from build123d import *

# Parameters (mm, degrees)
SKETCH1_W             = 198
SKETCH1_H             = 108
BOSS_EXTRUDE1_DEPTH   = 40
SKETCH4_W             = 181
SKETCH4_H             = 45
CUT_EXTRUDE2_DEPTH    = 10
CUT_EXTRUDE3_DEPTH    = 175
BOSS_EXTRUDE11_DEPTH  = 10
CUT_EXTRUDE12_DEPTH   = 175
CUT_EXTRUDE28_DEPTH   = 14.5
CUT_EXTRUDE29_DEPTH   = 14.5
CUT_EXTRUDE40_REACH   = 231.059
CUT_EXTRUDE5_DEPTH    = 23
SKETCH12_R            = 3.15
CUT_EXTRUDE9_DEPTH    = 230.058944379
SKETCH13_R            = 4.5
CUT_EXTRUDE10_DEPTH   = 16.5
SKETCH14_R            = 4.5
CUT_EXTRUDE11_DEPTH   = 16.5
SKETCH41_R            = 2.9
CUT_EXTRUDE21_DEPTH   = 7
CUT_EXTRUDE22_DEPTH   = 10
CUT_EXTRUDE23_DEPTH   = 10
CUT_EXTRUDE32_DEPTH   = 43.3
CUT_EXTRUDE34_DEPTH   = 55.4
CUT_EXTRUDE36_DEPTH   = 55.4
SKETCH90_R            = 6.1
CUT_EXTRUDE38_DEPTH   = 17
SKETCH96_R            = 2
CUT_EXTRUDE39_DEPTH   = 230.058944379
SKETCH98_R            = 7.5
CUT_EXTRUDE41_DEPTH   = 4
CORTAR_EXTRUIR1_DEPTH = 23
CORTAR_EXTRUIR2_DEPTH = 23


with BuildPart() as part:
    # Sketch1 → Boss-Extrude1 (new body)
    with BuildSketch(Plane(origin=(0, 0, 0), x_dir=(1, 0, 0), z_dir=(0, 1, 0))):
        with Locations((99, 54)):
            Rectangle(SKETCH1_W, SKETCH1_H)
    extrude(amount=BOSS_EXTRUDE1_DEPTH)

    # Sketch4 → Cut-Extrude2 (cut)
    with BuildSketch(Plane(origin=(0, 0, 0), x_dir=(1, 0, 0), z_dir=(0, 1, 0))):
        with Locations((99, 54)):
            Rectangle(SKETCH4_W, SKETCH4_H)
    extrude(amount=CUT_EXTRUDE2_DEPTH, mode=Mode.SUBTRACT)

    # Sketch5 → Cut-Extrude3 (cut)
    with BuildSketch(Plane(origin=(198, 0, 0), x_dir=(0, 0, -1), z_dir=(1, 0, 0))):
        Polygon((54, 40), (108, 28.52194567), (108, 40), align=None)
    extrude(amount=-CUT_EXTRUDE3_DEPTH, mode=Mode.SUBTRACT)

    # Sketch53 → Boss-Extrude11 (add)
    with BuildSketch(Plane(origin=(0, 10, 0), x_dir=(-1, 0, 0), z_dir=(0, -1, 0))):
        Polygon((-8.5, 51.5), (-8.5, 31.5), (-39.5, 31.5), align=None)
        Polygon((-8.5, 56.5), (-8.5, 76.5), (-39.5, 76.5), align=None)
        Polygon((-158.5, 76.5), (-189.5, 56.5), (-189.5, 76.5), align=None)
        Polygon((-158.5, 31.5), (-189.5, 51.5), (-189.5, 31.5), align=None)
    extrude(amount=BOSS_EXTRUDE11_DEPTH)

    # Sketch18 → Cut-Extrude12 (cut)
    with BuildSketch(Plane(origin=(198, 0, 0), x_dir=(0, 0, -1), z_dir=(1, 0, 0))):
        Polygon((0, 28.915391904), (0, 40), (54, 40), align=None)
    extrude(amount=-CUT_EXTRUDE12_DEPTH, mode=Mode.SUBTRACT)

    # Izq → Cut-Extrude28 (cut)
    with BuildSketch(Plane(origin=(0, 28.012686094, -12.204810084), x_dir=(1, 0, 0), z_dir=(0, 0.9167660546215654, -0.3994245874925693))):
        Polygon((8.5, 48.862182113), (29.5, 70.132603179), (8.5, 70.132603179), align=None)
    cut_extrude28 = extrude(amount=-CUT_EXTRUDE28_DEPTH, mode=Mode.SUBTRACT)

    # Der → Cut-Extrude29 (cut)
    with BuildSketch(Plane(origin=(0, -11.144923858, -4.62106599), x_dir=(1, 0, 0), z_dir=(0, 0.9237421135716327, 0.38301502270043264))):
        Polygon((8.5, 51.290217599), (29.5, 29.097876578), (8.5, 29.097876578), align=None)
    cut_extrude29 = extrude(amount=-CUT_EXTRUDE29_DEPTH, mode=Mode.SUBTRACT)

    # Cut-Extrude40: up to this face of the body (flat: up to its plane)
    cut_extrude40_end = Plane(part.part.faces().sort_by_distance((99, 10, -54))[0])
    # Sketch97 → Cut-Extrude40 (cut, up to the picked face)
    with BuildSketch(Plane(origin=(0, 0, 0), x_dir=(1, 0, 0), z_dir=(0, 1, 0)), mode=Mode.PRIVATE) as cut_extrude40_sk1:
        Polygon((8.5, 57.5), (29.5, 76.5), (158.5, 76.5), (189.5, 56.5), (189.5, 51.5), (158.5, 31.5), (29.5, 31.5), (8.5, 51.5), align=None)
    cut_extrude40_tool1 = split(extrude(cut_extrude40_sk1.sketch, amount=CUT_EXTRUDE40_REACH, mode=Mode.PRIVATE), bisect_by=cut_extrude40_end, keep=Keep.BOTH, mode=Mode.PRIVATE)
    cut_extrude40 = cut_extrude40_tool1.solids().sort_by(Axis((96.82024, 0, -54.014019), (0, 1, 0)))[0]
    add(cut_extrude40, mode=Mode.SUBTRACT)

    # Mirror2: Cut-Extrude28, Cut-Extrude29, Cut-Extrude40 across plane
    add(cut_extrude28.mirror(Plane(origin=(99, 0, 0), x_dir=(0, 0, 1), z_dir=(1, 0, 0))), mode=Mode.SUBTRACT)
    add(cut_extrude29.mirror(Plane(origin=(99, 0, 0), x_dir=(0, 0, 1), z_dir=(1, 0, 0))), mode=Mode.SUBTRACT)
    add(cut_extrude40.mirror(Plane(origin=(99, 0, 0), x_dir=(0, 0, 1), z_dir=(1, 0, 0))), mode=Mode.SUBTRACT)

    # Sketch7 → Cut-Extrude5 (cut)
    with BuildSketch(Plane(origin=(0, 0, 0), x_dir=(0, 0, -1), z_dir=(1, 0, 0))):
        Polygon((108, 40), (108, 35), (83.505102572, 40), align=None)
        Polygon((0, 35), (0, 40), (24.494897428, 40), align=None)
    extrude(amount=CUT_EXTRUDE5_DEPTH, mode=Mode.SUBTRACT)

    # Sketch12 → Cut-Extrude9 (cut, through all)
    with BuildSketch(Plane(origin=(0, 40, 0), x_dir=(1, 0, 0), z_dir=(0, 1, 0))):
        with Locations(Location((19.7, 98.85, 0), (0, 0, 270))):
            Circle(SKETCH12_R)
        with Locations(Location((99.7, 9.15, 0), (0, 0, 270))):
            Circle(SKETCH12_R)
        with Locations(Location((179.7, 9.15, 0), (0, 0, 270))):
            Circle(SKETCH12_R)
        with Locations(Location((19.7, 9.15, 0), (0, 0, 270))):
            Circle(SKETCH12_R)
        with Locations(Location((99.7, 98.85, 0), (0, 0, 270))):
            Circle(SKETCH12_R)
        with Locations(Location((179.7, 98.85, 0), (0, 0, 270))):
            Circle(SKETCH12_R)
    extrude(amount=-CUT_EXTRUDE9_DEPTH, mode=Mode.SUBTRACT)

    # Sketch13 → Cut-Extrude10 (cut)
    with BuildSketch(Plane(origin=(0, 49.252798516, -10.469005505), x_dir=(1, 0, 0), z_dir=(0, 0.9781476007338072, -0.20791169081775226))):
        with Locations(Location((46.5, 86.70989493, 0), (0, 0, 270))):
            Circle(SKETCH13_R)
        with Locations(Location((151.5, 86.70989493, 0), (0, 0, 270))):
            Circle(SKETCH13_R)
    extrude(amount=-CUT_EXTRUDE10_DEPTH, mode=Mode.SUBTRACT)

    # Sketch14 → Cut-Extrude11 (cut)
    with BuildSketch(Plane(origin=(0, 27.155811177, 8.572008905), x_dir=(1, 0, 0), z_dir=(0, 0.9795752495993454, 0.20107792114595804))):
        with Locations(Location((46.5, 22.974220944, 0), (0, 0, 270))):
            Circle(SKETCH14_R)
        with Locations(Location((151.5, 22.974220944, 0), (0, 0, 270))):
            Circle(SKETCH14_R)
    extrude(amount=-CUT_EXTRUDE11_DEPTH, mode=Mode.SUBTRACT)

    # Sketch41 → Cut-Extrude21 (cut)
    with BuildSketch(Plane(origin=(0, 0, 0), x_dir=(1, 0, 0), z_dir=(0, 1, 0))):
        with Locations(Location((139.5, 9, 0), (0, 0, 90))):
            Circle(SKETCH41_R)
        with Locations(Location((139.5, 99, 0), (0, 0, 90))):
            Circle(SKETCH41_R)
    extrude(amount=CUT_EXTRUDE21_DEPTH, mode=Mode.SUBTRACT)

    # Sketch42 → Cut-Extrude22 (cut)
    with BuildSketch(Plane.XY):
        with BuildLine():
            Line((142.3, 12.8), (152, 12.8))
            ThreePointArc((152, 12.8), (153.8, 11), (152, 9.2))
            Line((152, 9.2), (142.3, 9.2))
            ThreePointArc((142.3, 9.2), (140.5, 11), (142.3, 12.8))
        make_face()
    extrude(amount=-CUT_EXTRUDE22_DEPTH, mode=Mode.SUBTRACT)

    # Sketch43 → Cut-Extrude23 (cut)
    with BuildSketch(Plane(origin=(0, 0, -108), x_dir=(-1, 0, 0), z_dir=(0, 0, -1))):
        with BuildLine():
            Line((-55.7, 12.8), (-46, 12.8))
            ThreePointArc((-46, 12.8), (-44.2, 11), (-46, 9.2))
            Line((-46, 9.2), (-55.7, 9.2))
            ThreePointArc((-55.7, 9.2), (-57.5, 11), (-55.7, 12.8))
        make_face()
    extrude(amount=-CUT_EXTRUDE23_DEPTH, mode=Mode.SUBTRACT)

    # Sketch6 → Cut-Extrude32 (cut)
    with BuildSketch(Plane(origin=(0, 49.252798516, -10.469005505), x_dir=(1, 0, 0), z_dir=(0, 0.9781476007338072, -0.20791169081775226))):
        with BuildLine():
            Line((32.2, 72.70989493), (166.2, 72.70989493))
            ThreePointArc((166.2, 72.70989493), (168.321320344, 71.831215273), (169.2, 69.70989493))
            Line((169.2, 69.70989493), (169.2, 55.70989493))
            ThreePointArc((169.2, 55.70989493), (168.321320344, 53.588574586), (166.2, 52.70989493))
            Line((166.2, 52.70989493), (32.2, 52.70989493))
            ThreePointArc((32.2, 52.70989493), (30.078679656, 53.588574586), (29.2, 55.70989493))
            Line((29.2, 55.70989493), (29.2, 69.70989493))
            ThreePointArc((29.2, 69.70989493), (30.078679656, 71.831215273), (32.2, 72.70989493))
        make_face()
    extrude(amount=-CUT_EXTRUDE32_DEPTH, mode=Mode.SUBTRACT)

    # Sketch83 → Cut-Extrude34 (cut)
    with BuildSketch(Plane(origin=(0, 27.746275226, 5.695492352), x_dir=(1, 0, 0), z_dir=(0, 0.9795752495993454, 0.20107792114595804))):
        with BuildLine():
            Line((31.7, 52.814246893), (166.7, 52.814246893))
            ThreePointArc((166.7, 52.814246893), (168.467766953, 52.082013846), (169.2, 50.314246893))
            Line((169.2, 50.314246893), (169.2, 35.314246893))
            ThreePointArc((169.2, 35.314246893), (168.467766953, 33.54647994), (166.7, 32.814246893))
            Line((166.7, 32.814246893), (31.7, 32.814246893))
            ThreePointArc((31.7, 32.814246893), (29.932233047, 33.54647994), (29.2, 35.314246893))
            Line((29.2, 35.314246893), (29.2, 50.314246893))
            ThreePointArc((29.2, 50.314246893), (29.932233047, 52.082013846), (31.7, 52.814246893))
        make_face()
    extrude(amount=-CUT_EXTRUDE34_DEPTH, mode=Mode.SUBTRACT)

    # Sketch85 → Cut-Extrude36 (cut)
    with BuildSketch(Plane(origin=(0, 40, 0), x_dir=(1, 0, 0), z_dir=(0, 1, 0))):
        Polygon((0, 101.9), (6.1, 108), (0, 108), align=None)
        Polygon((0, 0), (6.1, 0), (0, 6.1), align=None)
        Polygon((198, 6.1), (191.9, 0), (198, 0), align=None)
        Polygon((198, 108), (191.9, 108), (198, 101.9), align=None)
    extrude(amount=-CUT_EXTRUDE36_DEPTH, mode=Mode.SUBTRACT)

    # Sketch90 → Cut-Extrude38 (cut)
    with BuildSketch(Plane(origin=(0, 40, 0), x_dir=(1, 0, 0), z_dir=(0, 1, 0))):
        with Locations(Location((19.7, 9.15, 0), (0, 0, 270))):
            Circle(SKETCH90_R)
        with Locations(Location((99.7, 9.15, 0), (0, 0, 270))):
            Circle(SKETCH90_R)
        with Locations(Location((179.7, 9.15, 0), (0, 0, 270))):
            Circle(SKETCH90_R)
        with Locations(Location((99.7, 98.85, 0), (0, 0, 270))):
            Circle(SKETCH90_R)
        with Locations(Location((179.7, 98.85, 0), (0, 0, 270))):
            Circle(SKETCH90_R)
        with Locations(Location((19.7, 98.85, 0), (0, 0, 270))):
            Circle(SKETCH90_R)
    extrude(amount=-CUT_EXTRUDE38_DEPTH, mode=Mode.SUBTRACT)

    # Sketch96 → Cut-Extrude39 (cut, through all)
    with BuildSketch(Plane(origin=(0, 0, 0), x_dir=(1, 0, 0), z_dir=(0, 1, 0))):
        with Locations(Location((15.45, 54, 0), (0, 0, 270))):
            Circle(SKETCH96_R)
        with Locations((185, 54)):
            Circle(SKETCH96_R)
    extrude(amount=CUT_EXTRUDE39_DEPTH, mode=Mode.SUBTRACT)

    # Sketch98 → Cut-Extrude41 (cut)
    with BuildSketch(Plane(origin=(0, 40, 0), x_dir=(1, 0, 0), z_dir=(0, 1, 0))):
        with Locations(Location((185, 54, 0), (0, 0, 270))):
            Circle(SKETCH98_R)
        with Locations(Location((15.45, 54, 0), (0, 0, 270))):
            Circle(SKETCH98_R)
    extrude(amount=-CUT_EXTRUDE41_DEPTH, mode=Mode.SUBTRACT)

    # Croquis1 → Cortar-Extruir1 (cut)
    with BuildSketch(Plane(origin=(0, 0, 0), x_dir=(0, 0, -1), z_dir=(1, 0, 0))):
        Polygon((108, 40), (108, 28.52194567), (54, 40), align=None)
    extrude(amount=CORTAR_EXTRUIR1_DEPTH, mode=Mode.SUBTRACT)

    # Croquis2 → Cortar-Extruir2 (cut)
    with BuildSketch(Plane(origin=(0, 0, 0), x_dir=(0, 0, -1), z_dir=(1, 0, 0))):
        Polygon((54, 40), (0, 40), (0, 28.915391904), align=None)
    extrude(amount=CORTAR_EXTRUIR2_DEPTH, mode=Mode.SUBTRACT)


solid = part.part
The model under review builds one solid part; all positions refer to its coordinate system, in mm. A direction names the side the tool comes from. Round coordinates to 2 decimals unless told otherwise and drop trailing zeros. Loops run counter-clockwise (first coordinate to the right, second up) from the corner with the lowest first, then second, coordinate; pieces in that order, holes last. Notation, with made-up numbers: (2.25, 22.5) -> (10.25, 22.5) arc R19 cw to (10.25, 47.5) -> close; hole circle Ø3 at (57.5, 21.25). An arc over 180 degrees is marked (long way). Return JSON: item names as keys, results as strings.
(1) Add section C-C on z = -37.5. Write out the cut boundary in (x, y).
Solved:
{"outline": "(0, 0) -> (8.5, 0) -> (8.5, 2.49) -> (23.2, 2.49) -> (23.2, 10) -> (29.2, 10) -> (29.2, 36.61) -> (0, 36.61) -> close; (169.2, 10) -> (174.8, 10) -> (174.8, 2.49) -> (189.5, 2.49) -> (189.5, 0) -> (198, 0) -> (198, 36.61) -> (169.2, 36.61) -> close"}
(2) The part is to be moulded in two halves that separate along Z. For faces 5 (the flat face through (147, 9.2, -5)), 6 (the flat face through (139, 7, -99)), 7 (the flat face through (100.386, 33.066, -86.622)), say which applies: released by +Z, released by -Z, zero draft, split by the parting line, or undercut.
Solved:
{"face 5": "zero draft", "face 6": "undercut", "face 7": "released by -Z"}
(3) Add section A-A on x = 179.7. State how many separate pieces and enclosed holes the cut face has, plus the area to 3 significant figures.
Solved:
{"separate pieces": "3", "enclosed holes": "0", "area": "2,910 mm2"}
(4) For line 1 (X direction, y = 28, z = -9); line 2 (Z direction, x = 139, y = 4); line 3 (X direction, y = 2, z = -9), list the stretches that pass through material, from the lowest coordinate up.
Solved:
{"line 1": "0 to 13.6, 25.8 to 93.6, 105.8 to 173.6, 185.8 to 198", "line 2": "-108 to -101.86, -96.14 to -76.5, -31.5 to -11.86, -6.14 to 0", "line 3": "0 to 16.55, 22.85 to 96.55, 102.85 to 136.6, 142.4 to 176.55, 182.85 to 198"}
(5) For faces 1 (the cylindrical face through (182.36, 11.66, -97.16)), 2 (the flat face through (169.2, 23, -69)), 3 (the flat face through (177, 23, -96)), 4 (the flat face through (99, 10, -54)), list the 3-axis set-ups (+Z, -Z, +X, -X, +Y, -Y) from which the entire face can be reached by the end or side of a thin tool; tool diameter is ignored.
Solved:
{"face 1": "+Y, -Y", "face 2": "none", "face 3": "+Y", "face 4": "-Y"}
(6) For pin 1 (8 mm diameter, centred on x = 50.5, z = -104.5, fed in from +Y); pin 2 (6 mm diameter, centred on x = 20, z = -10.5, fed in from +Y); pin 3 (5 mm diameter, centred on x = 139.5, z = -99, fed in from +Y); pin 4 (4 mm diameter, centred on x = 99.7, z = -9.15, fed in from -Y), all flat-tipped, find the tip position at first contact; note any pin that passes through.
Solved:
{"pin 1": "y = 30.12", "pin 2": "y = 23", "pin 3": "y = 30.97", "pin 4": "through"}
(7) Add section D-D on x = 76.5. Write out the cut boundary in (y, z), plus the area to 3 significant figures.
Solved:
{"outline": "(0, -108) -> (28.52, -108) -> (34.14, -81.59) -> (10, -76.46) -> (10, -76.5) -> (0, -76.5) -> close; (0, -31.5) -> (9.74, -31.5) -> (34.34, -26.45) -> (28.92, 0) -> (0, 0) -> close; (10, -56.01) -> (38.29, -62.03) -> (40, -54) -> (38.37, -46.04) -> (10, -51.86) -> close", "area": "2,190 mm2"}
